The model under review builds one solid part; all positions refer to its coordinate system, in mm. A direction names the side the tool comes from. Give positions to 0.01 mm unless a question says otherwise; leave off trailing zeros. Write item = value, one per line.
```python
from build123d import *

# Parameters (mm, degrees)
SKETCH2_R          = 4.725
CUT_EXTRUDE1_DEPTH = 7
SKETCH3_R          = 1.25
CUT_EXTRUDE2_DEPTH = 18.878835952
SKETCH4_R          = 2.5
CUT_EXTRUDE3_DEPTH = 14.878836
FILLET1_R          = 2


with BuildPart() as part:
    # Sketch1 → Revolve1 (revolve)
    with BuildSketch(Plane(origin=(0, 0, 0), x_dir=(1, 0, 0), z_dir=(0, 1, 0))):
        Polygon((11.693859716, 12.315), (11.693859716, 7), (14.693859716, 7), (13.193859716, 5), (14.693859716, 5), (16.193859716, 5), (16.193859716, 0), (-6.184976236, 0), (-6.184976236, 14.4), (8.993859716, 13.5), align=None)
    revolve(axis=Axis((-18.233766234, 0, 0), (1, 0, 0)))

    # Sketch2 → Cut-Extrude1 (cut)
    with BuildSketch(Plane.ZY.offset(6.184976236)):
        Circle(SKETCH2_R)
    extrude(amount=-CUT_EXTRUDE1_DEPTH, mode=Mode.SUBTRACT)

    # Sketch3 → Cut-Extrude2 (cut, through all)
    with BuildSketch(Plane(origin=(11.693859716, 0, 0), x_dir=(0, 0, -1), z_dir=(1, 0, 0))):
        with Locations((0, 10.5)):
            Circle(SKETCH3_R)
        with Locations((7.424621202, 7.424621202)):
            Circle(SKETCH3_R)
        with Locations((10.5, 0)):
            Circle(SKETCH3_R)
        with Locations((7.424621202, -7.424621202)):
            Circle(SKETCH3_R)
        with Locations((0, -10.5)):
            Circle(SKETCH3_R)
        with Locations((-7.424621202, -7.424621202)):
            Circle(SKETCH3_R)
        with Locations((-10.5, 0)):
            Circle(SKETCH3_R)
        with Locations((-7.424621202, 7.424621202)):
            Circle(SKETCH3_R)
    extrude(amount=-CUT_EXTRUDE2_DEPTH, mode=Mode.SUBTRACT)

    # Sketch4 → Cut-Extrude3 (cut)
    with BuildSketch(Plane.ZY.offset(6.184976236)):
        with Locations((0, 10.5)):
            Circle(SKETCH4_R)
        with Locations((7.424621202, 7.424621202)):
            Circle(SKETCH4_R)
        with Locations((10.5, 0)):
            Circle(SKETCH4_R)
        with Locations((7.424621202, -7.424621202)):
            Circle(SKETCH4_R)
        with Locations((0, -10.5)):
            Circle(SKETCH4_R)
        with Locations((-7.424621202, -7.424621202)):
            Circle(SKETCH4_R)
        with Locations((-10.5, 0)):
            Circle(SKETCH4_R)
        with Locations((-7.424621202, 7.424621202)):
            Circle(SKETCH4_R)
    extrude(amount=-CUT_EXTRUDE3_DEPTH, mode=Mode.SUBTRACT)

    # Fillet1
    fillet1_edges = [part.edges().sort_by_distance(p)[0] for p in [
        (16.193859716, 0, 5),
    ]]
    fillet(fillet1_edges, radius=FILLET1_R)


solid = part.part
```
1. Insertion check: P1, Ø5, axis at x = 5.5, y = -6, coming from the +Z side; P2, Ø2.5, axis at y = 0.5, z = 10.5, coming from the -X side; P3, Ø3, axis at x = 9, z = 10, coming from the -Y side; P4, Ø2, axis at y = -10.5, z = 0, coming from the +X side. Each pin has a flat end and moves straight along its axis. Give the tip position at first contact, or say it passes through.
Findings below:
P1 = 13.27
P2 = 8.69
P3 = -10.49
P4 = through
2. Draft analysis for pull direction Y (two halves, no side actions). For faces 4 (the flat face through (-6.185, 0, -7)), 5 (the cylindrical face through (13.215, -2.681, -6.466)), 6 (the flat face through (8.694, -6, 8)), state which applies: +Y half, -Y half, draft (parallel to the pull), parting line (faces both ways), or undercut.
Findings below:
face_4 = draft
face_5 = parting line
face_6 = undercut
3. Take a section at A-A on x = -1.5. Count the separate pieces of the cut face and the enclosed holes in it, and give its area (3 significant figures).
Findings below:
separate_pieces = 1
enclosed_holes = 9
area = 399 mm²
4. Machinability: for faces 1 (the flat face through (8.694, 9, -7)), 2 (the cylindrical face through (10.215, 6.316, -8.001)), 3 (the flat face through (11.694, -5.3, -5.3)), which of the approach directions +Z, -Z, +X, -X, +Y, -Y give a long, thin tool a straight path to every point of the face, cutting with its end or side? Answer none if there is none.
Findings below:
face_1 = -X
face_2 = +X, -X
face_3 = +X
5. For line 1 (Y direction, x = -1.75, z = 2.25); line 2 (Y direction, x = 8.5, z = -9.5); line 3 (Y direction, x = -3.5, z = -7.75), list the stretches that pass through material, from the lowest coordinate up. Write a range as from..to.
Findings below:
line_1 = -13.96..-11.59, -9.41..-4.15, 4.15..9.41, 11.59..13.96
line_2 = -9.63..-8.82, -6.03..-2.29, 2.29..6.03, 8.82..9.63
line_3 = -11.95..-9.9, -4.95..4.95, 9.9..11.95
